from build123d import *

# Parameters (mm, degrees)
ESQUISSE1_R        = 1.925
ESQUISSE1_R_2      = 0.925
ESQUISSE1_R_3      = 4
ESQUISSE1_R_4      = 4.5
BOSS_EXTRU_1_DEPTH = 5


with BuildPart() as part:
    # Esquisse1 → Boss.-Extru.1 (new body)
    with BuildSketch(Plane.XY):
        with BuildLine():
            ThreePointArc((-76.596505759, 7.891023923), (-88.219919815, -2.170080062), (-78.433932641, -14.026049982))
            ThreePointArc((-78.433932641, -14.026049982), (-4.607074536, -19.062713423), (69.387841086, -18.337855841))
            ThreePointArc((69.387841086, -18.337855841), (70.503800614, -18.28274944), (71.619694559, -18.226330568))
            ThreePointArc((71.619694559, -18.226330568), (88.178632292, 1.361410834), (67.556915532, 16.613388736))
            ThreePointArc((67.556915532, 16.613388736), (-4.256409128, 7.899259424), (-76.596505759, 7.891023923))
        make_face()
        with Locations((30.768040312, -3.82658336)):
            Circle(ESQUISSE1_R, mode=Mode.SUBTRACT)
        with Locations((-24.224638361, -4.723964207)):
            Circle(ESQUISSE1_R, mode=Mode.SUBTRACT)
        with Locations((77.721925672, -0.674275531)):
            Circle(ESQUISSE1_R_2, mode=Mode.SUBTRACT)
        with Locations((70.721925672, -7.674275531)):
            Circle(ESQUISSE1_R_2, mode=Mode.SUBTRACT)
        with Locations((63.721925672, -0.674275531)):
            Circle(ESQUISSE1_R_2, mode=Mode.SUBTRACT)
        with Locations((70.721925672, 6.325724469)):
            Circle(ESQUISSE1_R_2, mode=Mode.SUBTRACT)
        with Locations((70.721925672, -0.674275531)):
            Circle(ESQUISSE1_R_3, mode=Mode.SUBTRACT)
        with Locations((-77.258373302, -3.089045811)):
            Circle(ESQUISSE1_R_4, mode=Mode.SUBTRACT)
    extrude(amount=BOSS_EXTRU_1_DEPTH)


solid = part.part
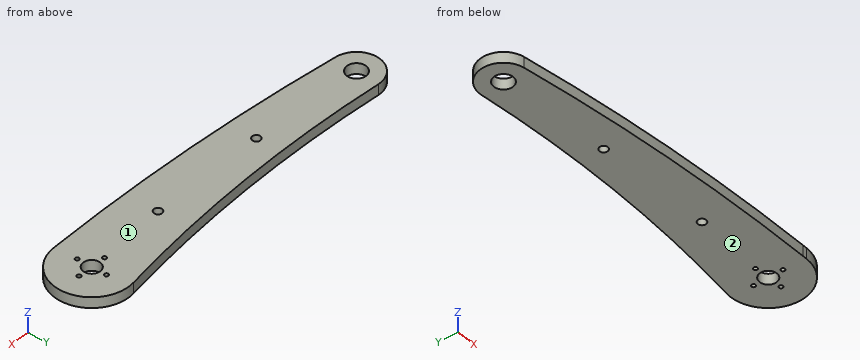
Part model, mm, in its own coordinate system. Face numbers are marked on the shaded views. Coordinates: 2 decimals unless noted, no trailing zeros. Write each loop counter-clockwise with the first axis right and the second up, starting at its lowest first coordinate (ties: lowest second). Pieces come first, ordered by that corner, then holes. Notation, with made-up numbers: (80, 33) - (130, 33) arc R29 cw to (130, 57) - close; hole circle Ø5 at (21, 28). An arc over 180 degrees is marked (long way). Put each result on its own line as item: value.
1. Two-plate mould, pull along Z, no slides. Class the marked faces 1 and 2: +Z half, -Z half, draft (parallel to the pull), parting line (faces both ways), or undercut.
Final values:
face 1: +Z half
face 2: -Z half
2. Band-saw the part on A-A (z = 2.2). Give the number of separate pieces and of enclosed holes in the cut face, then the cut area to 3 significant figures.
Final values:
separate pieces: 1
enclosed holes: 8
area: 4,620 mm²
3. Probe line 1 along X through (y, z) = (-5.5, 0.55); line 2 along X through (y, z) = (-6, 2.4); line 3 along Y through (x, z) = (-79.5, 1.15). List the from-to ranges inside material, lowest first. Write a range as [from, to].
Final values:
line 1: x = [-87.99, -81.06], [-73.46, -25.99], [-22.46, 29.82], [31.72, 87.62]
line 2: x = [-87.87, -80.69], [-73.83, -25.67], [-22.78, 87.47]
line 3: y = [-13.86, -6.99], [0.81, 7.68]
4. Flat gauge pins, fed straight in: pin 1 Ø3 at (y, z) = (-13, 4) entering from -X; pin 2 Ø1 at (x, z) = (65, 3) entering from +Y. Where does each tip first touch, or does it go through?
Final values:
pin 1: stops at x = -84.35
pin 2: stops at y = 16.24
5. Band-saw the part on B-B (x = -52). Write the cut outline in (y, z).
Final values:
outline: (-16.49, 0) - (6.91, 0) - (6.91, 5) - (-16.49, 5) - close
